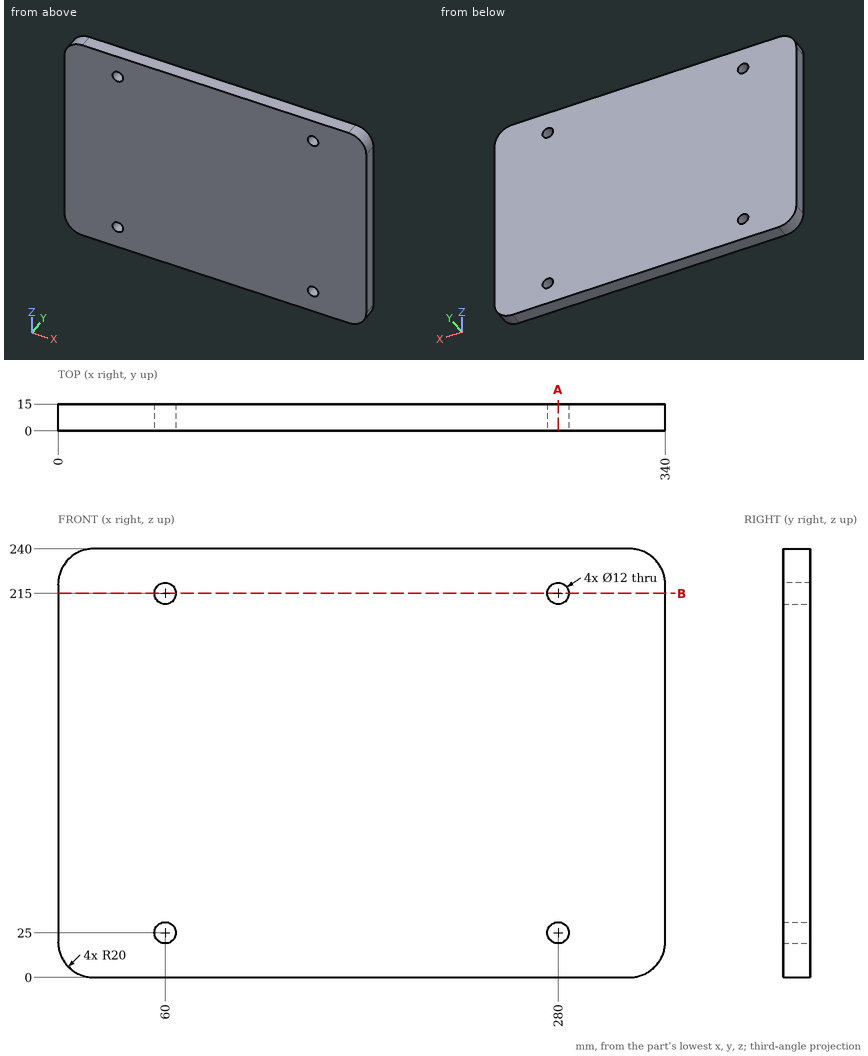
Could you check a few things on this drawing? It's one solid part, dimensions in mm from its lowest x, y, z. Give positions to 0.01 mm unless a question says otherwise; leave off trailing zeros. Order: outer loops, then holes, each group sorted by start corner. A loop starts at its lowest first (then second) coordinate and runs counter-clockwise, first axis right, second up.
1. Suppose I cut it at B-B (z = 215). Write out the boundary of the cut face in (x, y).
Answers below:
outline: (0, 0) - (54, 0) - (54, 15) - (0, 15) - close; (66, 0) - (274, 0) - (274, 15) - (66, 15) - close; (286, 0) - (340, 0) - (340, 15) - (286, 15) - close
2. I need wall thicknesses on L1, parallel to X at y = 11.75, z = 215; L2, parallel to Z at x = 280, y = 8.5; L3, parallel to Z at x = 320.5, y = 8.5. Which ranges of each line are inside material? Lowest first, please.
Answers below:
L1: x = 0 to 54, 66 to 274, 286 to 340
L2: z = 0 to 19, 31 to 209, 221 to 240
L3: z = 0.01 to 239.99
3. Suppose I cut it at A-A (x = 280). Write out the boundary of the cut face in (y, z).
Answers below:
outline: (0, 0) - (15, 0) - (15, 19) - (0, 19) - close; (0, 31) - (15, 31) - (15, 209) - (0, 209) - close; (0, 221) - (15, 221) - (15, 240) - (0, 240) - close
